Build history of the part. All positions in model axes, mm. Face numbers are marked on the shaded views. A direction names the side the tool comes from. Give positions to 0.01 mm unless a question says otherwise; leave off trailing zeros. One line per question, with ' | ' between items. Start each with the question number.
(1) Pull direction X, two halves, no side cores. Call the marked faces 1, 2, 3 and 4: +X half, -X half, draft (parallel to the pull), parting line (faces both ways), or undercut.
(2) Drill centre lines: L1, parallel to Z at x = 19.05, y = 7.5; L2, parallel to Z at x = -13.5, y = 6.75. Where is each one in solid material? Low to high. Write a range as from..to.
(3) Which spindle directions (+Z, -Z, +X, -X, +Y, -Y) get a long thin tool onto all of the face, cutting with end or side? Do the marked faces 5 and 6. Say none if no direction does.
(4) Pin check, flat tips, straight feed: pin 1 Ø0.5 at (y, z) = (12.5, -55) entering from -X; pin 2 Ø3 at (x, z) = (-26, -47) entering from +Y; pin 3 Ø3 at (x, z) = (0, 16) entering from +Y. Stop position of each tip, or through.
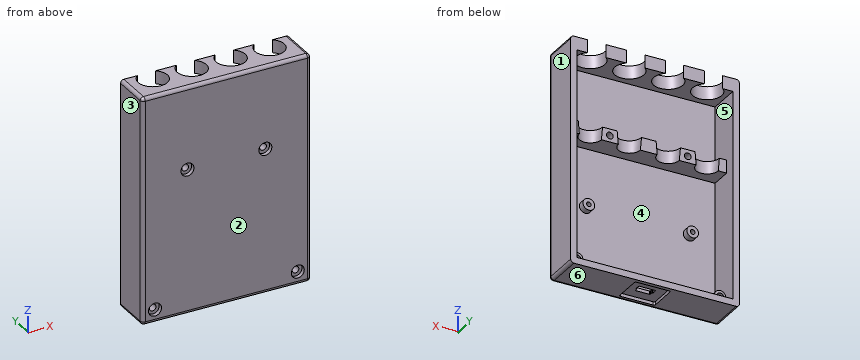
from build123d import *

# Parameters (mm, degrees)
SKETCH1_W                                       = 82.55
SKETCH1_H                                       = 111.125
BOSS_EXTRUDE1_DEPTH                             = 19.05
SKETCH14_W                                      = 76.2
SKETCH14_H                                      = 101.6
CUT_EXTRUDE3_DEPTH                              = 15.875
CUT_EXTRUDE4_REACH                              = 113.125
SKETCH11_R                                      = 7.1501
SKETCH17_R                                      = 2.778125
SKETCH17_W                                      = 76.2
SKETCH17_H                                      = 6.35
BOSS_EXTRUDE4_DEPTH                             = 10.3251
SKETCH18_R                                      = 5.953125
CUT_EXTRUDE5_DEPTH                              = 6.35
CUT_EXTRUDE5_TAPER                              = 5
CUT_EXTRUDE7_REACH                              = 113.125
FILLET6_R                                       = 1.5875
SKETCH19_R                                      = 2.8575
BOSS_EXTRUDE8_DEPTH                             = 3.175
CBORE_FOR_4_PAN_HEAD_MACHINE_SCREW3_D           = 3.2639
CBORE_FOR_4_PAN_HEAD_MACHINE_SCREW3_CBORE_D     = 6.35
CBORE_FOR_4_PAN_HEAD_MACHINE_SCREW3_CBORE_DEPTH = 2.032
F_4_40_TAPPED_HOLE1_D                           = 2.2606
F_4_40_TAPPED_HOLE1_DEPTH                       = 4.7752
F_4_40_TAPPED_HOLE1_TIP                         = 0.679152758
SKETCH39_W                                      = 17.4625
SKETCH39_H                                      = 14.2875
CUT_EXTRUDE8_DEPTH                              = 1.5875
FILLET7_R                                       = 0.79375
FILLET8_R                                       = 0.1984375
FILLET9_R                                       = 0.396875


with BuildPart() as part:
    # Sketch1 → Boss-Extrude1 (new body)
    with BuildSketch(Plane(origin=(0, 0, 0), x_dir=(1, 0, 0), z_dir=(0, 1, 0))):
        Rectangle(SKETCH1_W, SKETCH1_H)
    extrude(amount=BOSS_EXTRUDE1_DEPTH)

    # Sketch14 → Cut-Extrude3 (cut)
    with BuildSketch(Plane(origin=(0, 19.05, 0), x_dir=(-1, 0, 0), z_dir=(0, 1, 0))):
        with Locations((0, -1.5875)):
            Rectangle(SKETCH14_W, SKETCH14_H)
    extrude(amount=-CUT_EXTRUDE3_DEPTH, mode=Mode.SUBTRACT)

    # Sketch11 → Cut-Extrude4 (cut, up to next)
    with BuildSketch(Plane.XY.offset(55.5625), mode=Mode.PRIVATE) as cut_extrude4_sk1:
        with Locations((-28.575, 13.5001)):
            Circle(SKETCH11_R)
    cut_extrude4_tool1 = extrude(cut_extrude4_sk1.sketch, amount=-CUT_EXTRUDE4_REACH, mode=Mode.PRIVATE) & part.part
    add(cut_extrude4_tool1.solids().sort_by_distance((-28.575, 13.5001, 55.5625))[0], mode=Mode.SUBTRACT)
    # Sketch11 → Cut-Extrude4 (cut, up to next)
    with BuildSketch(Plane.XY.offset(55.5625), mode=Mode.PRIVATE) as cut_extrude4_sk2:
        with Locations((-9.525, 13.5001)):
            Circle(SKETCH11_R)
    cut_extrude4_tool2 = extrude(cut_extrude4_sk2.sketch, amount=-CUT_EXTRUDE4_REACH, mode=Mode.PRIVATE) & part.part
    add(cut_extrude4_tool2.solids().sort_by_distance((-9.525, 13.5001, 55.5625))[0], mode=Mode.SUBTRACT)
    # Sketch11 → Cut-Extrude4 (cut, up to next)
    with BuildSketch(Plane.XY.offset(55.5625), mode=Mode.PRIVATE) as cut_extrude4_sk3:
        with Locations((9.525, 13.5001)):
            Circle(SKETCH11_R)
    cut_extrude4_tool3 = extrude(cut_extrude4_sk3.sketch, amount=-CUT_EXTRUDE4_REACH, mode=Mode.PRIVATE) & part.part
    add(cut_extrude4_tool3.solids().sort_by_distance((9.525, 13.5001, 55.5625))[0], mode=Mode.SUBTRACT)
    # Sketch11 → Cut-Extrude4 (cut, up to next)
    with BuildSketch(Plane.XY.offset(55.5625), mode=Mode.PRIVATE) as cut_extrude4_sk4:
        with Locations((28.575, 13.5001)):
            Circle(SKETCH11_R)
    cut_extrude4_tool4 = extrude(cut_extrude4_sk4.sketch, amount=-CUT_EXTRUDE4_REACH, mode=Mode.PRIVATE) & part.part
    add(cut_extrude4_tool4.solids().sort_by_distance((28.575, 13.5001, 55.5625))[0], mode=Mode.SUBTRACT)

    # Sketch17 → Boss-Extrude4 (add)
    with BuildSketch(Plane(origin=(0, 3.175, 0), x_dir=(-1, 0, 0), z_dir=(0, 1, 0))):
        with Locations((34.925, -49.2125)):
            Circle(SKETCH17_R)
        with Locations((-34.925, -49.2125)):
            Circle(SKETCH17_R)
        with Locations((0, 15.08125)):
            Rectangle(SKETCH17_W, SKETCH17_H)
    extrude(amount=BOSS_EXTRUDE4_DEPTH)

    # Sketch18 → Cut-Extrude5 (cut)
    with BuildSketch(Plane.XY.offset(18.25625)):
        with Locations((-28.575, 13.5001)):
            Circle(SKETCH18_R)
        with Locations((-9.525, 13.5001)):
            Circle(SKETCH18_R)
        with Locations((9.525, 13.5001)):
            Circle(SKETCH18_R)
        with Locations((28.575, 13.5001)):
            Circle(SKETCH18_R)
    extrude(amount=-CUT_EXTRUDE5_DEPTH, taper=CUT_EXTRUDE5_TAPER, mode=Mode.SUBTRACT)

    # Sketch21 → Cut-Extrude7 (cut, up to next)
    with BuildSketch(Plane(origin=(0, 0, -55.5625), x_dir=(-1, 0, 0), z_dir=(0, 0, -1)), mode=Mode.PRIVATE) as cut_extrude7_sk1:
        Polygon((-3.683, 7.9375), (-3.683, 9.525), (-4.1671875, 9.525), (-4.1671875, 12.1046875), (4.1671875, 12.1046875), (4.1671875, 9.525), (3.683, 9.525), (3.683, 7.9375), align=None)
    cut_extrude7_tool1 = extrude(cut_extrude7_sk1.sketch, amount=-CUT_EXTRUDE7_REACH, mode=Mode.PRIVATE) & part.part
    add(cut_extrude7_tool1.solids().sort_by_distance((0, 10.08083, -55.5625))[0], mode=Mode.SUBTRACT)

    # Fillet6
    fillet6_edges = [part.edges().sort_by_distance(p)[0] for p in [
        (0, 0, 55.5625),
        (-41.275, 0, 0),
        (0, 0, -55.5625),
        (41.275, 0, 0),
        (41.275, 9.525, 55.5625),
        (-41.275, 9.525, 55.5625),
        (-41.275, 9.525, -55.5625),
        (41.275, 9.525, -55.5625),
    ]]
    fillet(fillet6_edges, radius=FILLET6_R)

    # Sketch19 → Boss-Extrude8 (add)
    with BuildSketch(Plane(origin=(0, 3.175, 0), x_dir=(-1, 0, 0), z_dir=(0, 1, 0))):
        with Locations((25.5143, -47.371)):
            Circle(SKETCH19_R)
        with Locations((-25.4, -47.3075)):
            Circle(SKETCH19_R)
        with Locations((25.4, -16.8275)):
            Circle(SKETCH19_R)
        with Locations((-25.4, -16.8275)):
            Circle(SKETCH19_R)
    extrude(amount=BOSS_EXTRUDE8_DEPTH)

    # CBORE for #4 Pan Head Machine Screw3 (through all)
    with Locations(Plane.XZ):
        with Locations((-19.05, 15.08125), (19.05, 15.08125), (-34.925, -49.2125), (34.925, -49.2125)):
            CounterBoreHole(CBORE_FOR_4_PAN_HEAD_MACHINE_SCREW3_D / 2, CBORE_FOR_4_PAN_HEAD_MACHINE_SCREW3_CBORE_D / 2, CBORE_FOR_4_PAN_HEAD_MACHINE_SCREW3_CBORE_DEPTH)

    # #4-40 Tapped Hole1
    with Locations(Plane(origin=(0, 6.35, 0), x_dir=(-1, 0, 0), z_dir=(0, 1, 0))):
        with Locations((25.5143, -47.371), (25.4, -16.8275), (-25.4, -16.8275), (-25.4, -47.3075)):
            Hole(F_4_40_TAPPED_HOLE1_D / 2, depth=F_4_40_TAPPED_HOLE1_DEPTH)
            with Locations((0, 0, -(F_4_40_TAPPED_HOLE1_DEPTH + F_4_40_TAPPED_HOLE1_TIP / 2))):  # 118° drill point
                Cone(0, F_4_40_TAPPED_HOLE1_D / 2, F_4_40_TAPPED_HOLE1_TIP, mode=Mode.SUBTRACT)

    # Sketch39 → Cut-Extrude8 (cut)
    with BuildSketch(Plane(origin=(0, 0, -55.5625), x_dir=(-1, 0, 0), z_dir=(0, 0, -1))):
        with Locations((0, 10.02109375)):
            Rectangle(SKETCH39_W, SKETCH39_H)
    extrude(amount=-CUT_EXTRUDE8_DEPTH, mode=Mode.SUBTRACT)

    # Fillet7
    fillet7_edges = [part.edges().sort_by_distance(p)[0] for p in [
        (-8.73125, 17.16484375, -54.76875),
        (-8.73125, 2.87734375, -54.76875),
        (8.73125, 2.87734375, -54.76875),
        (8.73125, 17.16484375, -54.76875),
    ]]
    fillet(fillet7_edges, radius=FILLET7_R)

    # Fillet8
    fillet8_edges = [part.edges().sort_by_distance(p)[0] for p in [
        (3.683, 9.525, -53.18125),
        (4.1671875, 9.525, -53.18125),
        (-4.1671875, 9.525, -53.18125),
        (-3.683, 9.525, -53.18125),
    ]]
    fillet(fillet8_edges, radius=FILLET8_R)

    # Fillet9
    fillet9_edges = [part.edges().sort_by_distance(p)[0] for p in [
        (-3.683, 7.9375, -53.18125),
        (3.683, 7.9375, -53.18125),
        (4.1671875, 12.1046875, -53.18125),
        (-4.1671875, 12.1046875, -53.18125),
    ]]
    fillet(fillet9_edges, radius=FILLET9_R)


solid = part.part
Result set:
1) face 1: +X half | face 2: draft | face 3: -X half | face 4: undercut
2) L1: z = -55.56..-52.39, 11.91..13.45, 16.71..18.26, 49.21..55.56 | L2: z = -55.56..-52.39, 11.91..18.26, 49.21..55.56
3) face 5: +Y | face 6: -Z, +X, -X, +Y, -Y
4) pin 1: stops at x = -41.07 | pin 2: stops at y = 6.35 | pin 3: stops at y = 13.5
